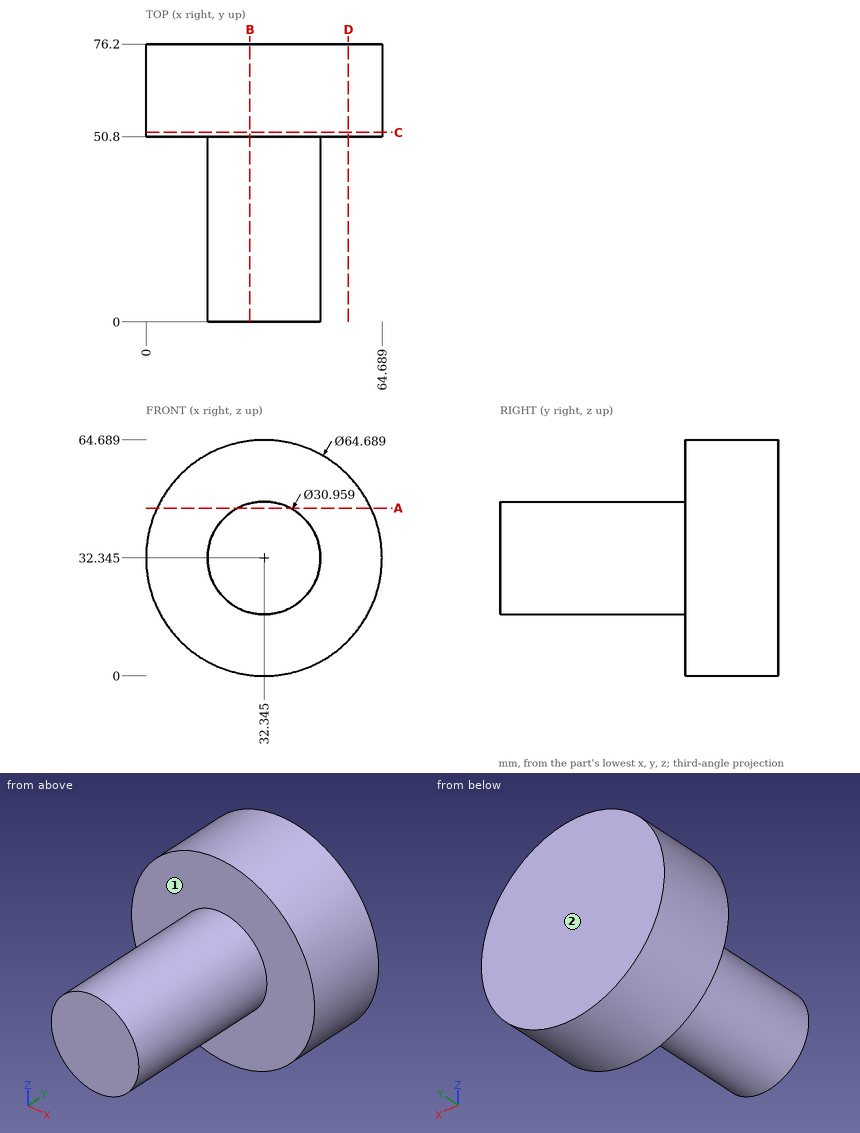
Verification items for this drawing (mm, ordinates from the low corner). A direction names the side the tool comes from. Round coordinates to 2 decimals unless told otherwise and drop trailing zeros. Loops run counter-clockwise (first coordinate to the right, second up) from the corner with the lowest first, then second, coordinate; pieces in that order, holes last. Notation, with made-up numbers: M 41.5,52 L 92.5,52 A17 ccw 92.5,78 Z; hole C 67.5,-30 d4. An arc over 180 degrees is marked long. Answer as a JSON object with one key per item and string values.
1. Gauge pin test, flat ends, axial feed: P1, Ø8, axis at x = 19.5, y = 31, coming from the -Z side; P2, Ø4, axis at y = 55.5, z = 9.5, coming from the -X side; P3, Ø3, axis at x = 26, z = 47.5, coming from the -Y side; P4, Ø1, axis at x = 19, y = 48.5, coming from the +Z side (1 decimal). Record the tip position at first contact, or that the pin passes through.
Reply:
{"P1": "stops at z = 19.64", "P2": "stops at x = 7.61", "P3": "stops at y = 0", "P4": "stops at z = 41"}
2. Section check D-D (x = 55.5). Record the boundary of the cut face in (y, z), plus the area to 3 significant figures.
Reply:
{"outline": "M 50.8,9.76 L 76.2,9.76 L 76.2,54.93 L 50.8,54.93 Z", "area": "1,150 mm²"}
3. Section check C-C (y = 52). Record the boundary of the cut face in (x, z) (1 decimal).
Reply:
{"outline": "C 32.3,32.3 d64.7"}
4. Section check A-A (z = 46). Record the boundary of the cut face in (x, y) (1 decimal), plus the area to 3 significant figures.
Reply:
{"outline": "M 3,50.8 L 25.1,50.8 L 25.1,0 L 39.6,0 L 39.6,50.8 L 61.7,50.8 L 61.7,76.2 L 3,76.2 Z", "area": "2,230 mm²"}
5. Scan lines: line 1 (Y direction, x = 22, z = 52); line 2 (X direction, y = 28, z = 33); line 3 (X direction, y = 60, z = 41). Record each from-to range of solid material in increasing order.
Reply:
{"line 1": "y = 50.8 to 76.2", "line 2": "x = 16.88 to 47.81", "line 3": "x = 1.18 to 63.51"}
6. Section check B-B (x = 28.5). Record the boundary of the cut face in (y, z).
Reply:
{"outline": "M 0,17.35 L 50.8,17.35 L 50.8,0.23 L 76.2,0.23 L 76.2,64.46 L 50.8,64.46 L 50.8,47.34 L 0,47.34 Z"}
7. Access from +Z, -Z, +X, -X, +Y, -Y to the whole of each face (thin tool, end or side, straight path). Record for the marked faces 1 and 2.
Reply:
{"face 1": "-Y", "face 2": "+Z, -Z, +X, -X, +Y"}
